Source: CAD feature listing. Evaluate the final solid. Frame: model axes, mm. Face numbers are marked on the shaded views. A direction names the side the tool comes from. Round coordinates to 2 decimals unless told otherwise and drop trailing zeros. Order: outer loops, then holes, each group sorted by start corner. A loop starts at its lowest first (then second) coordinate and runs counter-clockwise, first axis right, second up. Notation, with made-up numbers: (16.25, -34.5) -> (36.25, -34.5) arc R13 ccw to (36.25, -17.5) -> close; hole circle Ø1 at (-8.5, 3.5). An arc over 180 degrees is marked (long way). Answer as CSV lines item,"result". Start each with the question number.
(1) Contact query for flat-ended pins moving along their axis: P1, Ø5.5, axis at x = 0, y = -5, coming from the -Z side; P2, Ø11.5, axis at x = 0, z = 13, coming from the -Y side. Output: stop coordinate, or through.
(2) Section query C-C (x = 0). Output: boundary loops of the cut face in (y, z), plus the area to 3 significant figures.
(3) Pull-direction query (X, two-part tool) for the marked faces 3, 4, 5 and 6; classes: +X half, -X half, draft (parallel to the pull), parting line (faces both ways), or undercut.
(4) Section query D-D (y = -5). Output: boundary loops of the cut face in (x, z).
(5) Set-up query: the marked faces 1 and 2. Return all of +Z, -Z, +X, -X, +Y, -Y with unobstructed straight access to the full face (end or side cutting, diameter ignored); none if empty.
(6) Line query: line 1 along Y through (x, z) = (0, -3.5); line 2 along Z through (x, y) = (0, 13.5); line 3 along Y through (x, z) = (7, 21.5). Output: solid intervals per line, ascending. Write a range as from..to.
(7) Section query B-B (y = -1). Output: boundary loops of the cut face in (x, z).
(8) Section query A-A (z = 13). Output: boundary loops of the cut face in (x, y).
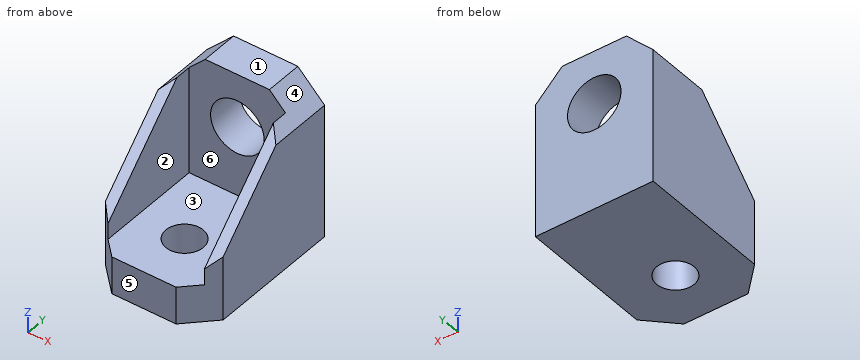
```python
from build123d import *

# Parameters (mm, degrees)
F0_W        = 2
F0_H        = 23
F0_W_2      = 18
F0_R        = 3.5
F1_DEPTH    = 7
F2_DEPTH    = 23
F3_R        = 5
F4_DEPTH    = 25
F5_SIZE     = 23
F6_T1_DEPTH = 32.7168298797
F6_T3_DEPTH = 32.7168298797


# Not quite as in the source:
# - a fillet or chamfer that OpenCascade refuses, or shapes differently, is made with other operations: its cross-section is extruded or revolved along the edge and cut away or added


with BuildPart() as f1:
    # F0 (on Top) → F1 (new body)
    with BuildSketch(Plane.XY):
        with Locations((-10, -3.5)):
            Rectangle(F0_W, F0_H)
        with Locations((0, -3.5)):
            Rectangle(F0_W_2, F0_H)
        with Locations((0, -5)):
            Circle(F0_R, mode=Mode.SUBTRACT)
        with Locations((10, -3.5)):
            Rectangle(F0_W, F0_H)
        Polygon((9, 8), (11, 8), (11, 15), (-11, 15), (-11, 8), (-9, 8), align=None)
    extrude(amount=-F1_DEPTH)

    # F0 (on Top) → F2 (join)
    with BuildSketch(Plane.XY):
        Polygon((9, 8), (11, 8), (11, 15), (-11, 15), (-11, 8), (-9, 8), align=None)
        with Locations((-10, -3.5)):
            Rectangle(F0_W, F0_H)
        with Locations((10, -3.5)):
            Rectangle(F0_W, F0_H)
    extrude(amount=F2_DEPTH)

    # F3 (on face) → F4 (cut)
    with BuildSketch(Plane.XZ.offset(-8)):
        with Locations((0, 13)):
            Circle(F3_R)
    extrude(amount=-F4_DEPTH, mode=Mode.SUBTRACT)

    # F5
    f5_edges = [f1.edges().sort_by_distance(p)[0] for p in [
        (10, -15, 23),
        (-10, -15, 23),
    ]]
    chamfer(f5_edges, length=F5_SIZE)

    # F6: chamfer of 5 on 4 edges, made by hand

    # F6_s2 → F6_t1 (cut)
    with BuildSketch(Plane.XY.offset(-19.8584149398)):
        Polygon((-6, -15), (-11, -10), (-11, -15), align=None)
        Polygon((6, -15), (11, -10), (11, -15), align=None)
    extrude(amount=F6_T1_DEPTH, mode=Mode.SUBTRACT)

    # F6_s4 → F6_t3 (cut)
    with BuildSketch(Plane.XZ.offset(-27.8584149398)):
        Polygon((-11, 18), (-6, 23), (-11, 23), align=None)
        Polygon((11, 18), (6, 23), (11, 23), align=None)
    extrude(amount=F6_T3_DEPTH, mode=Mode.SUBTRACT)


solid = f1.part
```
Answer block:
1,P1,"through"
1,P2,"y = 8"
2,outline,"(-15, -7) -> (-8.5, -7) -> (-8.5, 0) -> (-15, 0) -> close; (-1.5, -7) -> (15, -7) -> (15, 8) -> (8, 8) -> (8, 0) -> (-1.5, 0) -> close; (8, 18) -> (15, 18) -> (15, 23) -> (8, 23) -> close"
2,area,"252 mm2"
3,face 3,"undercut"
3,face 4,"+X half"
3,face 5,"draft"
3,face 6,"undercut"
4,outline,"(-11, -7) -> (-3.5, -7) -> (-3.5, 0) -> (-9, 0) -> (-9, 10) -> (-11, 10) -> close; (3.5, -7) -> (11, -7) -> (11, 10) -> (9, 10) -> (9, 0) -> (3.5, 0) -> close"
5,face 1,"+Z, +X, -X, +Y, -Y"
5,face 2,"+Z, -Y"
6,line 1,"-15..-8.5, -1.5..15"
6,line 2,"-7..8, 18..23"
6,line 3,"8..15"
7,outline,"(-11, -7) -> (11, -7) -> (11, 14) -> (9, 14) -> (9, 0) -> (-9, 0) -> (-9, 14) -> (-11, 14) -> close"
8,outline,"(-11, -2) -> (-9, -2) -> (-9, 8) -> (-5, 8) -> (-5, 15) -> (-11, 15) -> close; (5, 8) -> (9, 8) -> (9, -2) -> (11, -2) -> (11, 15) -> (5, 15) -> close"
